Read the model definition and answer for the solid it produces. Units are mm, in the model's axes. Face numbers are marked on the shaded views. A direction names the side the tool comes from. Coordinates: 2 decimals unless noted, no trailing zeros. Write each loop counter-clockwise with the first axis right and the second up, starting at its lowest first coordinate (ties: lowest second). Pieces come first, ordered by that corner, then holes. Notation, with made-up numbers: M 83.25,30.25 L 101.25,30.25 A14 cw 101.25,53.25 Z; hole C 40.5,-4.5 d6. An arc over 180 degrees is marked long. Use a Markdown table: item, result. Add a question column.
from build123d import *

# Parameters (mm, degrees)
CHAMFER_1_SIZE      = 0.5
CUT_EXTRUDE_START   = -7
SKETCH_2_R          = 12.139773641
CUT_EXTRUDE_1_DEPTH = 7


with BuildPart() as part:
    # Эскиз1 → Повернуть1 (revolve)
    with BuildSketch(Plane.XY, mode=Mode.PRIVATE) as revolve_1_sk:
        Polygon((0, 77.5), (-5, 77.5), (-5, 17.5), (-9.5, 17.5), (-9.5, 10.5), (-5, 10.5), (-5, 10), (-10, 10), (-19, 5), (-19, 0), (-5, 0), (-5, 7), (0, 7), align=None)
    revolve(revolve_1_sk.sketch.rotate(Axis((0, 0, 0), (0, 1, 0)), 180), axis=Axis((0, 0, 0), (0, 1, 0)))  # turned: the seam where the file's is

    # Фаска1
    chamfer_1_edges = [part.edges().sort_by_distance(p)[0] for p in [
        (-5, 77.5, 0),
    ]]
    chamfer(chamfer_1_edges, length=CHAMFER_1_SIZE)

    # Эскиз2 → Вырез-Вытянуть1 (cut)
    with BuildSketch(Plane(origin=(0, 17.5, 0), x_dir=(1, 0, 0), z_dir=(0, 1, 0)).offset(CUT_EXTRUDE_START)):
        Circle(SKETCH_2_R)
        Polygon((0, 9.5), (-8.227241336, 4.75), (-8.227241336, -4.75), (0, -9.5), (8.227241336, -4.75), (8.227241336, 4.75), align=None, mode=Mode.SUBTRACT)
    extrude(amount=CUT_EXTRUDE_1_DEPTH, mode=Mode.SUBTRACT)


solid = part.part
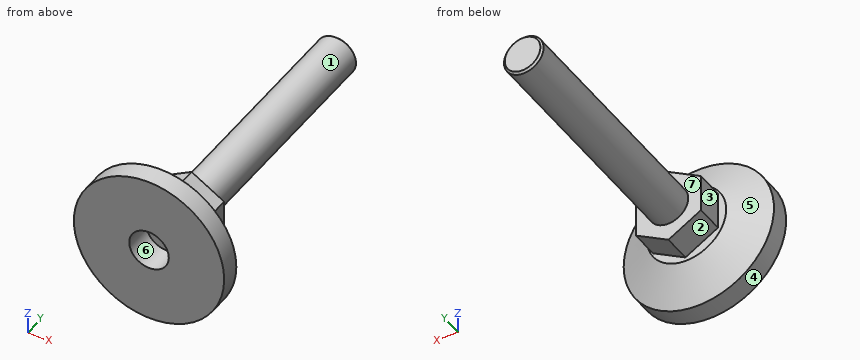
Item 1: Find section B-B on y = 44. Give the vertices of the cut face in (x, z), then the cut area to 3 significant figures.
Item 2: Determine the mould class of the marked faces 5, 6 and 7 for opening direction X: pulls with the +X half, pulls with the -X half, needs draft (parallel to the pull), parting line crosses it, or undercut.
Item 3: Each of these flat-tipped pins is pushed along its axis until it touches: pin 1 (3 mm diameter, centred on x = 1, z = 1, fed in from -Y); pin 2 (10 mm diameter, centred on y = 59.5, z = -8.5, fed in from +X); pin 3 (6 mm diameter, centred on y = 9, z = -10.5, fed in from -X); pin 4 (13 mm diameter, centred on x = -2.5, z = -0.5, fed in from -Y). Where does it stop, or does it pass through?
Item 4: For the marked faces 1, 2, 3 and 4, determine the directions among +Z, -Z, +X, -X, +Y, -Y from which every point of the face is accessible in a straight line to the end or side of a thin tool.
Item 5: Consider probe 1 along Y at (x, z) = (-4.5, -4.5); probe 2 along Z at (x, y) = (0, 4); probe 3 along Y at (x, z) = (1, 0). Determine where each line is inside the solid, lowest interval first.
Item 6: Find section A-A on z = 0. Give the vertices of the cut face in (x, y).
Geometry says:
| question | item | result |
|---|---|---|
| 1 | outline | C 0,0 d10 |
| 1 | area | 78.5 mm2 |
| 2 | face 5 | parting line crosses it |
| 2 | face 6 | undercut |
| 2 | face 7 | needs draft |
| 3 | pin 1 | stops at y = 7 |
| 3 | pin 2 | stops at x = 3.57 |
| 3 | pin 3 | stops at x = -13.97 |
| 3 | pin 4 | stops at y = 0 |
| 4 | face 1 | +Y |
| 4 | face 2 | -Z, -X, +Y |
| 4 | face 3 | +Z, -Z, -X, +Y |
| 4 | face 4 | +Y, -Y |
| 5 | probe 1 | y = 0 to 10, 10.5 to 17.5 |
| 5 | probe 2 | z = -19 to -5, 5 to 19 |
| 5 | probe 3 | y = 7 to 77.5 |
| 6 | outline | M -19,0 L -5,0 L -5,7 L 5,7 L 5,0 L 19,0 L 19,5 L 10,10 L 5,10 L 5,10.5 L 8.23,10.5 L 8.23,17.5 L 5,17.5 L 5,77 L 4.5,77.5 L -4.5,77.5 L -5,77 L -5,17.5 L -8.23,17.5 L -8.23,10.5 L -5,10.5 L -5,10 L -10,10 L -19,5 Z |
